Work out the finished part from the listing and answer in its coordinate system (mm). Face numbers are marked on the shaded views. Coordinates: 2 decimals unless noted, no trailing zeros. Loops run counter-clockwise (first coordinate to the right, second up) from the corner with the lowest first, then second, coordinate; pieces in that order, holes last. Notation, with made-up numbers: (-38.75, 31.25) -> (16.25, 31.25) arc R34 ccw to (16.25, 63.25) -> close; hole circle Ø2 at (44.5, 29). An arc over 180 degrees is marked (long way). Answer as CSV lines item,"result".
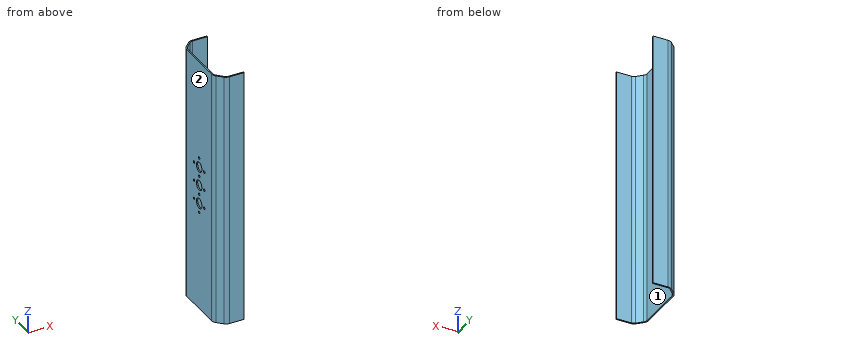
```python
from build123d import *

# Parameters (mm, degrees)
BOSS_EXTRU_1_DEPTH      = 204
ESQUISSE2_R             = 4
ESQUISSE2_R_2           = 1
ENL_V_MAT_EXTRU_1_DEPTH = 22


with BuildPart() as part:
    # Esquisse1 → Boss.-Extru.1 (new body)
    with BuildSketch(Plane.XY):
        with BuildLine():
            Line((-1.464466094, 1.464466094), (-5.606601718, 5.606601718))
            ThreePointArc((-5.606601718, 5.606601718), (-6.690465474, 7.228718462), (-7.071067812, 9.142135624))
            Line((-7.071067812, 9.142135624), (-7.071067812, 45.857864376))
            ThreePointArc((-7.071067812, 45.857864376), (-6.690465474, 47.771281538), (-5.606601718, 49.393398282))
            Line((-5.606601718, 49.393398282), (-1.464466094, 53.535533906))
            ThreePointArc((-1.464466094, 53.535533906), (0.15765065, 54.619397663), (2.071067812, 55))
            Line((2.071067812, 55), (13.928932188, 55))
            Line((13.928932188, 55), (13.928932188, 54))
            Line((13.928932188, 54), (2.071067812, 54))
            ThreePointArc((2.071067812, 54), (0.540334082, 53.69551813), (-0.757359313, 52.828427125))
            Line((-0.757359313, 52.828427125), (-4.899494937, 48.686291501))
            ThreePointArc((-4.899494937, 48.686291501), (-5.766585942, 47.388598106), (-6.071067812, 45.857864376))
            Line((-6.071067812, 45.857864376), (-6.071067812, 9.142135624))
            ThreePointArc((-6.071067812, 9.142135624), (-5.766585942, 7.611401894), (-4.899494937, 6.313708499))
            Line((-4.899494937, 6.313708499), (-0.757359313, 2.171572875))
            ThreePointArc((-0.757359313, 2.171572875), (0.540334082, 1.30448187), (2.071067812, 1))
            Line((2.071067812, 1), (13.928932188, 1))
            Line((13.928932188, 1), (13.928932188, 0))
            Line((13.928932188, 0), (2.071067812, 0))
            ThreePointArc((2.071067812, 0), (0.15765065, 0.380602337), (-1.464466094, 1.464466094))
        make_face()
    extrude(amount=BOSS_EXTRU_1_DEPTH)

    # Esquisse2 → Enlèv. mat.-Extru.1 (cut, through all)
    with BuildSketch(Plane.ZY.offset(7.071067812)):
        with Locations((102, 27.5)):
            Circle(ESQUISSE2_R)
        with Locations((102, 35)):
            Circle(ESQUISSE2_R_2)
        with Locations((109.5, 27.5)):
            Circle(ESQUISSE2_R_2)
        with Locations((102, 20)):
            Circle(ESQUISSE2_R_2)
        with Locations((94.5, 27.5)):
            Circle(ESQUISSE2_R_2)
        with Locations((117, 27.5)):
            Circle(ESQUISSE2_R)
        with Locations((117, 35)):
            Circle(ESQUISSE2_R_2)
        with Locations((124.5, 27.5)):
            Circle(ESQUISSE2_R_2)
        with Locations((117, 20)):
            Circle(ESQUISSE2_R_2)
        with Locations((87, 27.5)):
            Circle(ESQUISSE2_R)
        with Locations((87, 35)):
            Circle(ESQUISSE2_R_2)
        with Locations((87, 20)):
            Circle(ESQUISSE2_R_2)
        with Locations((79.5, 27.5)):
            Circle(ESQUISSE2_R_2)
    extrude(amount=-ENL_V_MAT_EXTRU_1_DEPTH, mode=Mode.SUBTRACT)


solid = part.part
```
(1) A cutting plane is placed at B-B, the plane z = 42. Write down the section's boundary in (x, y).
Computed values:
outline,"(-7.07, 9.14) arc R5 ccw to (-5.61, 5.61) -> (-1.46, 1.46) arc R5 ccw to (2.07, 0) -> (13.93, 0) -> (13.93, 1) -> (2.07, 1) arc R4 cw to (-0.76, 2.17) -> (-4.9, 6.31) arc R4 cw to (-6.07, 9.14) -> (-6.07, 45.86) arc R4 cw to (-4.9, 48.69) -> (-0.76, 52.83) arc R4 cw to (2.07, 54) -> (13.93, 54) -> (13.93, 55) -> (2.07, 55) arc R5 ccw to (-1.46, 53.54) -> (-5.61, 49.39) arc R5 ccw to (-7.07, 45.86) -> close"
(2) Flat-ended cylindrical pins translate along their axes: pin 1 Ø1.6 at (y, z) = (35, 102) entering from -X; pin 2 Ø2.5 at (y, z) = (20, 87) entering from +X. Find the tip coordinate at first contact, or state that the pin passes through.
Computed values:
pin 1,"through"
pin 2,"x = -6.07"
(3) For a pull along Y with two mould halves and no side action, classify the marked faces 1 and 2 as pulls with the +Y half, pulls with the -Y half, needs draft (parallel to the pull), parting line crosses it, or undercut.
Computed values:
face 1,"undercut"
face 2,"needs draft"
(4) Consider line 1 along Y through (x, z) = (-6.25, 87); line 2 along Y through (x, z) = (-6.45, 102); line 3 along Y through (x, z) = (10.5, 159.5). Determine where each line is inside the solid, lowest interval first.
Computed values:
line 1,"6.4 to 19, 21 to 23.5, 31.5 to 34, 36 to 48.6"
line 2,"6.73 to 19, 21 to 23.5, 31.5 to 34, 36 to 48.27"
line 3,"0 to 1, 54 to 55"
(5) A cutting plane is placed at A-A, the plane x = 4.5. Write down the section's boundary in (y, z), and give its area (3 significant figures).
Computed values:
outline,"(0, 0) -> (1, 0) -> (1, 204) -> (0, 204) -> close; (54, 0) -> (55, 0) -> (55, 204) -> (54, 204) -> close"
area,"408 mm2"
